```python
from build123d import *

# Parameters (mm, degrees)
BOSS_EXTRUDE1_DEPTH      = 30
SKETCH11_R               = 44.958564256
BOSS_EXTRUDE2_DEPTH      = 120
CUT_EXTRUDE1_DEPTH       = 163.940010531
SKETCH20_R               = 1.7
CUT_EXTRUDE13_DEPTH      = 24
SKETCH22_R               = 1.7
CUT_EXTRUDE14_DEPTH      = 24
SKETCH23_R               = 1.7
CUT_EXTRUDE15_DEPTH      = 24
CUT_EXTRUDE21_START      = -70
CUT_EXTRUDE21_DEPTH      = 70
CUT_EXTRUDE22_DEPTH      = 70
CIRPATTERN1_START        = 80
CIRPATTERN1_DEPTH        = 70
CHAMFER1_SIZE            = 4
SKETCH37_R               = 1.7
CUT_EXTRUDE23_DEPTH      = 177.933966729
CUT_EXTRUDE24_DEPTH      = 177.95016312
CUT_EXTRUDE24_DEPTH_BACK = 177.95016312
CUT_EXTRUDE25_DEPTH      = 177.95016312
CUT_EXTRUDE25_DEPTH_BACK = 177.95016312
SKETCH39_R               = 1.7


# Read off the part's stored shape, not the designer's step: CirPattern1
with BuildPart() as part:
    # Sketch2 → Boss-Extrude1 (new body)
    with BuildSketch(Plane(origin=(0, 0, 0), x_dir=(1, 0, 0), z_dir=(0, 1, 0))):
        with BuildLine():
            Line((-33.044792054, -32.835258764), (-11.913772202, -45.035258764))
            Line((-11.913772202, -45.035258764), (-11.497954912, -43.463427532))
            ThreePointArc((-11.497954912, -43.463427532), (0.991222154, -44.947635963), (13.402827335, -42.914295048))
            ThreePointArc((13.402827335, -42.914295048), (32.384657539, -31.185035772), (43.389409835, -11.77419272))
            Line((43.389409835, -11.77419272), (44.958564256, -12.2))
            Line((44.958564256, -12.2), (44.958564256, 12.2))
            Line((44.958564256, 12.2), (43.389409835, 11.77419272))
            ThreePointArc((43.389409835, 11.77419272), (38.393686215, 23.392249973), (30.359999068, 33.159356999))
            ThreePointArc((30.359999068, 33.159356999), (10.7465178, 43.655295843), (-11.497954912, 43.463427532))
            Line((-11.497954912, 43.463427532), (-11.913772202, 45.035258764))
            Line((-11.913772202, 45.035258764), (-33.044792054, 32.835258764))
            Line((-33.044792054, 32.835258764), (-31.891454922, 31.689234812))
            ThreePointArc((-31.891454922, 31.689234812), (-39.458623491, 21.547378777), (-43.899995544, 9.698602542))
            ThreePointArc((-43.899995544, 9.698602542), (-43.177821403, -12.527898422), (-31.891454922, -31.689234812))
            Line((-31.891454922, -31.689234812), (-33.044792054, -32.835258764))
        make_face()
    extrude(amount=BOSS_EXTRUDE1_DEPTH)

    # Sketch11 → Boss-Extrude2 (add)
    with BuildSketch(Plane(origin=(0, 30, 0), x_dir=(1, 0, 0), z_dir=(0, 1, 0))):
        with Locations(Location((0, 0, 0), (0, 0, 104.817769832))):
            Circle(SKETCH11_R)
    extrude(amount=BOSS_EXTRUDE2_DEPTH)

    # Sketch3 → Cut-Extrude1 (cut, through all)
    with BuildSketch(Plane(origin=(0, 0, 0), x_dir=(-1, 0, 0), z_dir=(0, -1, 0))):
        Polygon((21.650635095, 12.5), (0, 25), (-21.650635095, 12.5), (-21.650635095, -12.5), (0, -25), (21.650635095, -12.5), align=None)
    extrude(amount=-CUT_EXTRUDE1_DEPTH, mode=Mode.SUBTRACT)

    # Sketch20 → Cut-Extrude13 (cut)
    with BuildSketch(Plane(origin=(44.958564256, 0, 0), x_dir=(0, 0, -1), z_dir=(1, 0, 0))):
        with Locations((-6.75, 8.5)):
            Circle(SKETCH20_R)
        with Locations((6.75, 8.5)):
            Circle(SKETCH20_R)
    extrude(amount=-CUT_EXTRUDE13_DEPTH, mode=Mode.SUBTRACT)

    # Sketch22 → Cut-Extrude14 (cut)
    with BuildSketch(Plane(origin=(-22.479282128, 0, -38.935258764), x_dir=(-0.8660254037844386, 0, 0.5000000000000003), z_dir=(-0.5000000000000002, 0, -0.8660254037844385))):
        with Locations((6.75, 8.5)):
            Circle(SKETCH22_R)
        with Locations((-6.75, 8.5)):
            Circle(SKETCH22_R)
    extrude(amount=-CUT_EXTRUDE14_DEPTH, mode=Mode.SUBTRACT)

    # Sketch23 → Cut-Extrude15 (cut)
    with BuildSketch(Plane(origin=(-22.479282128, 0, 38.935258764), x_dir=(0.8660254037844386, 0, 0.5), z_dir=(-0.5000000000000001, 0, 0.8660254037844387))):
        with Locations((-6.75, 8.5)):
            Circle(SKETCH23_R)
        with Locations((6.75, 8.5)):
            Circle(SKETCH23_R)
    extrude(amount=-CUT_EXTRUDE15_DEPTH, mode=Mode.SUBTRACT)

    # Sketch35 → Cut-Extrude21 (cut)
    with BuildSketch(Plane(origin=(0, 150, 0), x_dir=(1, 0, 0), z_dir=(0, 1, 0)).offset(CUT_EXTRUDE21_START)):
        with BuildLine():
            Line((-37.366729854, 25), (-37.366729854, -25))
            ThreePointArc((-37.366729854, -25), (-44.958564256, 0), (-37.366729854, 25))
        make_face()
    extrude(amount=CUT_EXTRUDE21_DEPTH, mode=Mode.SUBTRACT)

    # Sketch36 → Cut-Extrude22 (cut)
    with BuildSketch(Plane(origin=(0, 150, 0), x_dir=(1, 0, 0), z_dir=(0, 1, 0))):
        Polygon((-26, 26), (-26, 0), (-26, -26), (0, -26), (26, -26), (26, 0), (26, 26), (0, 26), align=None)
    extrude(amount=-CUT_EXTRUDE22_DEPTH, mode=Mode.SUBTRACT)

    # CirPattern1 outline → CirPattern1 (cut)
    with BuildSketch(Plane(origin=(0, 0, 0), x_dir=(1, 0, 0), z_dir=(0, 1, 0)).offset(CIRPATTERN1_START)):
        with BuildLine():
            Line((25, -37.366729854), (-25, -37.366729854))
            ThreePointArc((-25, -37.366729854), (0, -44.958564256), (25, -37.366729854))
        make_face()
        with BuildLine():
            ThreePointArc((25, 37.366729854), (0, 44.958564256), (-25, 37.366729854))
            Line((-25, 37.366729854), (25, 37.366729854))
        make_face()
        with BuildLine():
            Line((37.366729854, 25), (37.366729854, -25))
            ThreePointArc((37.366729854, -25), (44.958564256, 0), (37.366729854, 25))
        make_face()
    extrude(amount=CIRPATTERN1_DEPTH, mode=Mode.SUBTRACT)

    # Chamfer1
    chamfer1_edges = [part.edges().sort_by_distance(p)[0] for p in [
        (-26, 115, -26),
        (26, 115, -26),
        (26, 115, 26),
        (-26, 115, 26),
    ]]
    chamfer(chamfer1_edges, length=CHAMFER1_SIZE)

    # Sketch37 → Cut-Extrude23 (cut, through all)
    with BuildSketch(Plane.ZY.offset(37.366729854)):
        with Locations(Location((-17, 138, 0), (0, 0, 180))):
            Circle(SKETCH37_R)
        with Locations(Location((-17, 92, 0), (0, 0, 180))):
            Circle(SKETCH37_R)
        with Locations(Location((17, 92, 0), (0, 0, 180))):
            Circle(SKETCH37_R)
        with Locations(Location((17, 138, 0), (0, 0, 180))):
            Circle(SKETCH37_R)
    extrude(amount=-CUT_EXTRUDE23_DEPTH, mode=Mode.SUBTRACT)

    # Sketch38 → Cut-Extrude24 (cut, two sides: drawn at the far end of the back side and taken through both)
    with BuildSketch(Plane(origin=(0, 0, -37.366729854), x_dir=(-1, 0, 0), z_dir=(0, 0, -1)).offset(-CUT_EXTRUDE24_DEPTH_BACK)):
        Polygon((-25, 150), (25.064026091, 150), (25, 115), (-25, 115), align=None)
    extrude(amount=CUT_EXTRUDE24_DEPTH + CUT_EXTRUDE24_DEPTH_BACK, mode=Mode.SUBTRACT)

    # Sketch39 → Cut-Extrude25 (cut, two sides: drawn at the far end of the back side and taken through both)
    with BuildSketch(Plane(origin=(0, 0, -37.366729854), x_dir=(-1, 0, 0), z_dir=(0, 0, -1)).offset(-CUT_EXTRUDE25_DEPTH_BACK)):
        with Locations((-17, 97.5)):
            Circle(SKETCH39_R)
        with Locations((17, 97.5)):
            Circle(SKETCH39_R)
    extrude(amount=CUT_EXTRUDE25_DEPTH + CUT_EXTRUDE25_DEPTH_BACK, mode=Mode.SUBTRACT)


solid = part.part
```
Model file for the job. Use its own axes, mm. A direction names the side the tool comes from. Coordinates: 2 decimals unless noted, no trailing zeros. Order: outer loops, then holes, each group sorted by start corner. A loop starts at its lowest first (then second) coordinate and runs counter-clockwise, first axis right, second up. Notation, with made-up numbers: M 35.5,-39 L 72.5,-39 A23 ccw 72.5,-14 Z; hole C 31,80 d1. An arc over 180 degrees is marked long. Answer as CSV lines item,"result".
(1) 3-axis set-ups, long thin cutter, end or side, ignore diameter. For faces 5 (the cylindrical face through (33.47, 6.84, -6.38)), 6 (the flat face through (10.67, 39.44, -18.84)), 7 (the flat face through (0, 98, -26)), 8 (the flat face through (0, 115, -32)), 9 (the flat face through (40, 80, 0)): which of +Z, -Z, +X, -X, +Y, -Y reach the whole face in a straight line?
Geometry says:
face 5,"+X"
face 6,"+Y, -Y"
face 7,"+Y"
face 8,"+Z, -Z, +Y"
face 9,"+Z, -Z, +X, +Y"
(2) Wall check: line 1 along Y through (x, z) = (33, -17); line 2 along Y through (x, z) = (17, -33); line 3 along X through (y, z) = (96, 19). Give the ranges that are in metal, low to high.
Geometry says:
line 1,"y = 0 to 90.3, 93.7 to 136.3, 139.7 to 150"
line 2,"y = 0 to 95.8, 99.2 to 115"
line 3,"x = -37.37 to -26, 26 to 37.37"
(3) Pull direction Z, two halves, no side cores. Call faces 1 (the flat face through (-40, 80, 0)), 2 (the cylindrical face through (33.47, 6.84, 7.12)), 3 (the flat face through (-24, 100, -24)), 4 (the flat face through (0, 97, 37.367)): +Z half, -Z half, draft (parallel to the pull), parting line (faces both ways), or undercut.
Geometry says:
face 1,"draft"
face 2,"undercut"
face 3,"undercut"
face 4,"+Z half"
(4) Band-saw the part on B-B, the plane x = 10. List the corners of the cut face in (y, z), then the cut area to 3 significant figures.
Geometry says:
outline,"M 0,-43.83 L 80,-43.83 L 80,-37.37 L 115,-37.37 L 115,-26 L 80,-26 L 80,-19.23 L 0,-19.23 Z; M 0,19.23 L 80,19.23 L 80,26 L 115,26 L 115,37.37 L 80,37.37 L 80,43.83 L 0,43.83 Z"
area,"4,730 mm2"
(5) Band-saw the part on C-C, the plane z = -6.75. List the corners of the cut face in (x, y).
Geometry says:
outline,"M -44.45,0 L -21.65,0 L -21.65,80 L -26,80 L -26,150 L -37.37,150 L -37.37,80 L -44.45,80 Z; M 21.65,0 L 44.96,0 L 44.96,6.8 L 21.65,6.8 Z; M 21.65,10.2 L 44.96,10.2 L 44.96,30 L 44.45,30 L 44.45,80 L 37.37,80 L 37.37,150 L 26,150 L 26,80 L 21.65,80 Z"
(6) Band-saw the part on D-D, the plane y = 14. List the corners of the cut face in (x, z), then the cut area to 3 significant figures.
Geometry says:
outline,"M -33.04,-32.84 L -11.91,-45.04 L -11.5,-43.46 A44.96 ccw 43.39,-11.77 L 44.96,-12.2 L 44.96,12.2 L 43.39,11.77 A44.96 ccw -11.5,43.46 L -11.91,45.04 L -33.04,32.84 L -31.89,31.69 A44.96 ccw -31.89,-31.69 Z; hole M -21.65,-12.5 L 0,-25 L 21.65,-12.5 L 21.65,12.5 L 0,25 L -21.65,12.5 Z"
area,"4,760 mm2"
(7) Flat gauge pins, fed straight in: pin 1 (15 mm diameter, centred on y = 112, z = -5.5, fed in from -X); pin 2 (4 mm diameter, centred on y = 92, z = -17, fed in from +X); pin 3 (1 mm diameter, centred on x = 2, y = 53, fed in from -Z). Where does each tip first touch, or does it go through?
Geometry says:
pin 1,"stops at x = -37.37"
pin 2,"stops at x = 37.37"
pin 3,"stops at z = -44.93"
(8) Band-saw the part on A-A, the plane y = 97.5. State how many separate pieces and enclosed holes the cut face has, then the cut area to 3 significant figures.
Geometry says:
separate pieces,"4"
enclosed holes,"0"
area,"2,490 mm2"
